Geometry check sheet. Reference: the model listing, model coordinates, mm. Face numbers are marked on the shaded views. A direction names the side the tool comes from. Round coordinates to 2 decimals unless told otherwise and drop trailing zeros. Write each loop counter-clockwise with the first axis right and the second up, starting at its lowest first coordinate (ties: lowest second). Pieces come first, ordered by that corner, then holes. Notation, with made-up numbers: (23, -20.5) -> (76, -20.5) arc R26 cw to (76, 13.5) -> close; hole circle Ø5 at (68.5, -12). An arc over 180 degrees is marked (long way). Return JSON: item names as keys, results as strings. Group by question number.
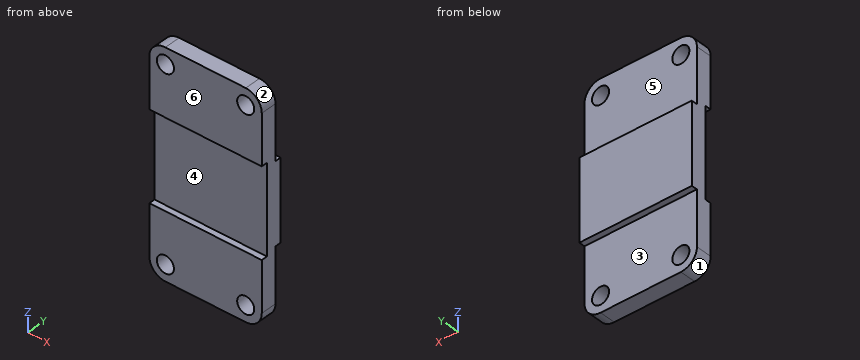
Autodesk Inventor part; units mm, degrees
ref_plane "YZ Plane" through (0, 0, 0) normal (1, 0, 0) x (0, 1, 0)
ref_plane "XZ Plane" through (0, 0, 0) normal (0, 1, 0) x (-1, 0, 0)
ref_plane "XY Plane" through (0, 0, 0) normal (0, 0, 1) x (1, 0, 0)
sketch "Boceto1" plane through (0, 0, 0) normal (0, 1, 0) x (-1, 0, 0)
  line L0 (-20, 55) -> (20, 55)
  line L1 (28, 47) -> (28, -47)
  line L2 (20, -55) -> (-20, -55)
  line L3 (-28, -47) -> (-28, 47)
  line L4 (-28, 55) -> (28, -55) construction
  line L5 (28, 55) -> (-28, -55) construction
  arc A0 (28, 47) -> (20, 55) centre (20, 47) ccw
  arc A1 (20, -55) -> (28, -47) centre (20, -47) ccw
  arc A2 (-28, -47) -> (-20, -55) centre (-20, -47) ccw
  arc A3 (-20, 55) -> (-28, 47) centre (-20, 47) ccw
  circle A4 centre (20, 47) radius 4.25
  circle A5 centre (-20, 47) radius 4.25
  circle A6 centre (20, -47) radius 4.25
  circle A7 centre (-20, -47) radius 4.25
  line L6 (-28, 20) -> (28, 20)
  line L7 (28, 20) -> (28, -20)
  line L8 (28, -20) -> (-28, -20)
  line L9 (-28, -20) -> (-28, 20)
  line L10 (-28, 20) -> (28, -20) construction
  line L11 (28, 20) -> (-28, -20) construction
  point P0 (0, 0)
  dimension "d0" = 56
  dimension "d1" = 110
  dimension "d2" = 8
  dimension "d3" = 8.5
  dimension "d4" = 8.5
  dimension "d5" = 8.5
  dimension "d6" = 8.5
  dimension "d7" = 56
  dimension "d8" = 40
extrude "Extrusión1" add sketch "Boceto1" along normal blind 8 contours L0 A0 L1 L6 L3 A3 | L8 L1 A1 L2 A2 L3
extrude "Extrusión2" add sketch "Boceto1" along normal blind 11 contours L6 L1 L8 L3
sketch "Boceto2" plane through (28, 0, 47) normal (1, 0, 0) x (0, 0, -1)
  line L0 (25, 3) -> (69, 3)
  line L1 (69, 3) -> (69, 0)
  line L2 (69, 0) -> (25, 0)
  line L3 (25, 0) -> (25, 3)
  line L4 (0, 0) -> (94, 0)
  point P0 (47, 0)
  point P1 (47, 0)
  dimension "d13" = 44
  dimension "d14" = 3
extrude "Extrusión3" cut sketch "Boceto2" against normal through all
properties part number "Base polea"
1) Material ranges on probe 1 along Z at (x, y) = (20, 4.75); probe 2 along Z at (x, y) = (1, 1.5); probe 3 along Z at (x, y) = (21, 7.5), recorded low to high. Write a range as [from, to].
2) Mould release check, pull along Z, two halves, no side actions. Record for the marked faces 1, 2, 3 and 4: +Z half, -Z half, draft (parallel to the pull), parting line (faces both ways), or undercut.
3) Sectioned sample at D-D on z = 44.5. Enter the section's corners in (x, y).
4) Sectioned sample at C-C on y = 7. Enter the section's corners in (x, z).
5) Go/stop test with flat-tipped pins: P1, Ø13, axis at x = -2, z = 4.5, coming from the -Y side; P2, Ø17.5, axis at x = -12, z = -30.5, coming from the +Y side; P3, Ø2.5, axis at x = -12, y = 9.5, coming from the -Z side. Record where each tip stops, or that it passes through.
6) Sectioned sample at B-B on x = 22. Enter the section's corners in (y, z), and give its area (3 significant figures).
7) Sectioned sample at A-A on y = 1.25. Enter the section's corners in (x, z), and give its area (3 significant figures).
8) Tool access check on the marked faces 5 and 6. Record the directions out of +Z, -Z, +X, -X, +Y, -Y that give a thin tool (end or side, any length) a straight path to the whole face; none if there is none.
Evaluation:
{
 "1": {"probe 1": "z = [-55, -51.25], [-42.75, 42.75], [51.25, 55]", "probe 2": "z = [-55, -22], [22, 55]", "probe 3": "z = [-54.94, -51.13], [-42.87, 42.87], [51.13, 54.94]"},
 "2": {"face 1": "-Z half", "face 2": "+Z half", "face 3": "draft", "face 4": "undercut"},
 "3": {"outline": "(-28, 0) -> (-23.44, 0) -> (-23.44, 8) -> (-28, 8) -> close; (-16.56, 0) -> (16.56, 0) -> (16.56, 8) -> (-16.56, 8) -> close; (23.44, 0) -> (28, 0) -> (28, 8) -> (23.44, 8) -> close"},
 "4": {"outline": "(-28, -47) arc R8 ccw to (-20, -55) -> (20, -55) arc R8 ccw to (28, -47) -> (28, 47) arc R8 ccw to (20, 55) -> (-20, 55) arc R8 ccw to (-28, 47) -> close; hole circle Ø8.5 at (-20, -47); hole circle Ø8.5 at (-20, 47); hole circle Ø8.5 at (20, -47); hole circle Ø8.5 at (20, 47)"},
 "5": {"P1": "stops at y = 3", "P2": "stops at y = 8", "P3": "stops at z = -20"},
 "6": {"outline": "(0, -54.75) -> (8, -54.75) -> (8, -50.75) -> (0, -50.75) -> close; (0, -43.25) -> (8, -43.25) -> (8, -20) -> (11, -20) -> (11, 20) -> (8, 20) -> (8, 43.25) -> (0, 43.25) -> (0, 22) -> (3, 22) -> (3, -22) -> (0, -22) -> close; (0, 50.75) -> (8, 50.75) -> (8, 54.75) -> (0, 54.75) -> close", "area": "744 mm2"},
 "7": {"outline": "(-28, -47) arc R8 ccw to (-20, -55) -> (20, -55) arc R8 ccw to (28, -47) -> (28, -22) -> (-28, -22) -> close; (-28, 22) -> (28, 22) -> (28, 47) arc R8 ccw to (20, 55) -> (-20, 55) arc R8 ccw to (-28, 47) -> close; hole circle Ø8.5 at (-20, -47); hole circle Ø8.5 at (-20, 47); hole circle Ø8.5 at (20, -47); hole circle Ø8.5 at (20, 47)", "area": "3,410 mm2"},
 "8": {"face 5": "+Z, +X, -X, +Y", "face 6": "+Z, -Z, +X, -X, -Y"}
}
